Read the model definition and answer for the solid it produces. Units are mm, in the model's axes. Face numbers are marked on the shaded views. A direction names the side the tool comes from. Coordinates: 2 decimals unless noted, no trailing zeros. Loops run counter-clockwise (first coordinate to the right, second up) from the corner with the lowest first, then second, coordinate; pieces in that order, holes last. Notation, with made-up numbers: M 46.25,14 L 70.25,14 A10 ccw 70.25,19 Z; hole C 72.5,-33.5 d7. An arc over 180 degrees is marked long. Use one line per item in the form item = value. Start each with the question number.
1. The part is cut by section A-A (x = 0). Give the vertices of the cut face in (y, z).
2. A tool of negligible diameter and unlimited length cuts with its end or side. For the marked faces 1 and 2, from which of +Z, -Z, +X, -X, +Y, -Y can it reach the whole face along a straight path? Write none if from no direction.
3. Flat-ended cylindrical pins translate along their axes: pin 1 (10 mm diameter, centred on y = 17, z = -5, fed in from -X); pin 2 (2 mm diameter, centred on y = 37.5, z = -2.5, fed in from -X); pin 3 (2 mm diameter, centred on x = 6, y = 26, fed in from +Z). Find the tip coordinate at first contact, or state that the pin passes through.
4. Find the intervals of material crossed by probe 1 along Y at (x, z) = (0.5, -7.75); probe 2 along Z at (x, y) = (-6.5, 14); probe 3 along Z at (x, y) = (0.5, 58.5), in increasing order. Write a range as [from, to].
5. The part is cut by section B-B (y = 54.5). Give the vertices of the cut face in (x, z).
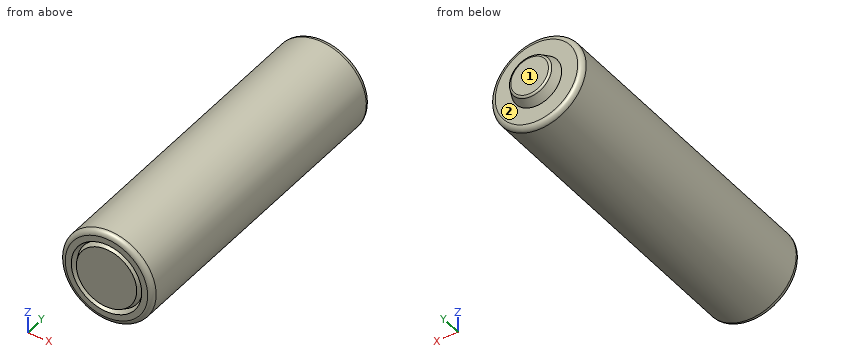
from build123d import *

# Parameters (mm, degrees)
SKETCH1_R           = 9.2
BOSS_EXTRUDE1_DEPTH = 63
SKETCH2_R           = 4.997387286
BOSS_EXTRUDE2_DEPTH = 2
BOSS_EXTRUDE2_TAPER = 25
SKETCH3_R           = 7.00167494
SKETCH3_R_2         = 6.004433393
CUT_EXTRUDE1_DEPTH  = 3
CUT_EXTRUDE1_TAPER  = 25
FILLET1_R           = 1
FILLET2_R           = 0.5
FILLET3_R           = 1


with BuildPart() as part:
    # Sketch1 → Boss-Extrude1 (new body)
    with BuildSketch(Plane(origin=(0, 0, 0), x_dir=(1, 0, 0), z_dir=(0, 1, 0))):
        with Locations(Location((0, 0, 0), (0, 0, 270))):
            Circle(SKETCH1_R)
    extrude(amount=BOSS_EXTRUDE1_DEPTH)

    # Sketch2 → Boss-Extrude2 (add)
    with BuildSketch(Plane(origin=(0, 63, 0), x_dir=(1, 0, 0), z_dir=(0, 1, 0))):
        Circle(SKETCH2_R)
    extrude(amount=BOSS_EXTRUDE2_DEPTH, taper=BOSS_EXTRUDE2_TAPER)

    # Sketch3 → Cut-Extrude1 (cut)
    with BuildSketch(Plane.XZ):
        Circle(SKETCH3_R)
        Circle(SKETCH3_R_2, mode=Mode.SUBTRACT)
    extrude(amount=-CUT_EXTRUDE1_DEPTH, taper=CUT_EXTRUDE1_TAPER, mode=Mode.SUBTRACT)

    # Fillet1
    fillet1_edges = [part.edges().sort_by_distance(p)[0] for p in [
        (0, 63, -9.2),
    ]]
    fillet(fillet1_edges, radius=FILLET1_R)

    # Fillet2
    fillet2_edges = [part.edges().sort_by_distance(p)[0] for p in [
        (-4.064771969, 65, 0),
    ]]
    fillet(fillet2_edges, radius=FILLET2_R)

    # Fillet3
    fillet3_edges = [part.edges().sort_by_distance(p)[0] for p in [
        (0, 0, -9.2),
    ]]
    fillet(fillet3_edges, radius=FILLET3_R)


solid = part.part
Computed values:
q1.outline = M 0,-8.2 A1 ccw 1,-9.2 L 62,-9.2 A1 ccw 63,-8.2 L 63,-5 L 64.71,-4.2 A0.5 ccw 65,-3.75 L 65,3.75 A0.5 ccw 64.71,4.2 L 63,5 L 63,8.2 A1 ccw 62,9.2 L 1,9.2 A1 ccw 0,8.2 L 0,7 L 1.07,6.5 L 0,6 L 0,-6 L 1.07,-6.5 L 0,-7 Z
q2.face_1 = +Z, -Z, +X, -X, +Y
q2.face_2 = +Y
q3.pin_1 = -9.2
q3.pin_2 = -9.08
q3.pin_3 = 7.72
q4.probe_1 = [0, 63]
q4.probe_2 = [-6.51, 6.51]
q4.probe_3 = [-9.19, 9.19]
q5.outline = C 0,0 d18.4
